Work out the finished part from the listing and answer in its coordinate system (mm). Face numbers are marked on the shaded views. A direction names the side the tool comes from. Coordinates: 2 decimals unless noted, no trailing zeros. Order: outer loops, then holes, each group sorted by start corner. A loop starts at its lowest first (then second) coordinate and runs counter-clockwise, first axis right, second up. Notation, with made-up numbers: M 19,-25 L 66,-25 A21 cw 66,13 Z; hole C 35.25,-33.5 d11. An arc over 180 degrees is marked long. Use a Markdown table: item, result.
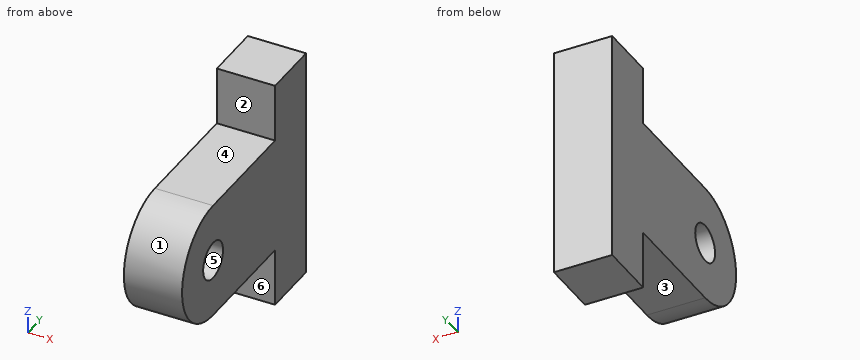
from build123d import *

# Parameters (mm, degrees)
SKETCH_3_R      = 1.6
EXTRUDE_1_DEPTH = 5


with BuildPart() as part:
    # 草图3 → 凸台-拉伸1 (new body)
    with BuildSketch(Plane(origin=(0, 0, 0), x_dir=(0, 0, -1), z_dir=(1, 0, 0))):
        with BuildLine():
            Line((0, 0), (20, 0))
            Line((20, 0), (20, -5))
            Line((20, -5), (15, -5))
            Line((15, -5), (15, -15))
            ThreePointArc((15, -15), (10, -20), (5, -15))
            Line((5, -15), (5, -5))
            Line((5, -5), (0, -5))
            Line((0, -5), (0, 0))
        make_face()
        with Locations((10, -15)):
            Circle(SKETCH_3_R, mode=Mode.SUBTRACT)
    extrude(amount=EXTRUDE_1_DEPTH)


solid = part.part
(1) A cutting plane is placed at B-B (x = 3.05). Determine the outline of the cut face in (y, z).
Conclusion:
| item | result |
|---|---|
| outline | M -15,-15 L -5,-15 L -5,-20 L 0,-20 L 0,0 L -5,0 L -5,-5 L -15,-5 A5 ccw Z; hole C -15,-10 d3.2 |
(2) Determine the mould class of the marked faces 4, 5 and 6 for opening direction Y: pulls with the +Y half, pulls with the -Y half, needs draft (parallel to the pull), parting line crosses it, or undercut.
Conclusion:
| item | result |
|---|---|
| face 4 | needs draft |
| face 5 | undercut |
| face 6 | pulls with the -Y half |
(3) Given P1, Ø2.5, axis at x = 3, z = -16.5, coming from the -Y side; P2, Ø1.5, axis at x = 2, z = -7, coming from the -Y side; P3, Ø1.5, axis at x = 3.5, y = -12.5, coming from the -Z side, each flat-ended and moving along its own axis, determine where each tip first touches the part or whether it passes through.
Conclusion:
| item | result |
|---|---|
| P1 | y = -5 |
| P2 | y = -19.47 |
| P3 | z = -15 |
(4) Straight lines are drawn through the part: L1, parallel to Y at x = 2.2, z = -10; L2, parallel to Y at x = 2.4, z = -2; L3, parallel to Z at x = 0.4, y = -12. For each, find the intervals that lie inside material, in ascending order.
Conclusion:
| item | result |
|---|---|
| L1 | -20 to -16.6, -13.4 to 0 |
| L2 | -5 to 0 |
| L3 | -15 to -5 |
(5) A cutting plane is placed at C-C (y = -12). Determine the outline of the cut face in (x, z).
Conclusion:
| item | result |
|---|---|
| outline | M 0,-15 L 5,-15 L 5,-5 L 0,-5 Z |
(6) A cutting plane is placed at A-A (z = -10). Determine the outline of the cut face in (x, y).
Conclusion:
| item | result |
|---|---|
| outline | M 0,-20 L 5,-20 L 5,-16.6 L 0,-16.6 Z; M 0,-13.4 L 5,-13.4 L 5,0 L 0,0 Z |
(7) A cutting plane is placed at D-D (z = -4.5). Determine the outline of the cut face in (x, y).
Conclusion:
| item | result |
|---|---|
| outline | M 0,-5 L 5,-5 L 5,0 L 0,0 Z |
(8) Which of the six approach directions +Z, -Z, +X, -X, +Y, -Y give full straight-line access (tool end or side, diameter ignored) to the marked faces 1, 2 and 3?
Conclusion:
| item | result |
|---|---|
| face 1 | +X, -X, -Y |
| face 2 | +Z, +X, -X, -Y |
| face 3 | -Z, +X, -X, -Y |
